Geometry: final body of the model. Coordinates: model frame, mm. Coordinates: 2 decimals unless noted, no trailing zeros. Order: outer loops, then holes, each group sorted by start corner. A loop starts at its lowest first (then second) coordinate and runs counter-clockwise, first axis right, second up. Notation, with made-up numbers: (71, 12) -> (88, 12) arc R33 cw to (88, 44) -> close; hole circle Ø9 at (1.5, -38.5). An arc over 180 degrees is marked (long way). Use one line per item in the form item = value.
```python
from build123d import *

# Parameters (mm, degrees)
SKETCH_1_W      = 23
SKETCH_1_H      = 4.3
EXTRUDE_1_DEPTH = 0.6


with BuildPart() as part:
    # Эскиз1 → Бобышка-Вытянуть1 (new body)
    with BuildSketch(Plane.XY):
        with BuildLine():
            Line((0, 0), (56, 0))
            Line((56, 0), (56, 15.7))
            Line((56, 15.7), (15, 15.7))
            ThreePointArc((15, 15.7), (10.112556238, 5.353927161), (0, 0))
        make_face()
        with Locations((37.5, 7.85)):
            Rectangle(SKETCH_1_W, SKETCH_1_H, mode=Mode.SUBTRACT)
    extrude(amount=EXTRUDE_1_DEPTH)


solid = part.part
```
1) Section C-C, the plane y = 7. Output: boundary loops of the cut face in (x, z), and give its area (3 significant figures).
Results found:
outline = (11.51, 0) -> (26, 0) -> (26, 0.6) -> (11.51, 0.6) -> close; (49, 0) -> (56, 0) -> (56, 0.6) -> (49, 0.6) -> close
area = 12.9 mm2
2) Section A-A, the plane z = 0.5. Output: boundary loops of the cut face in (x, y).
Results found:
outline = (0, 0) -> (56, 0) -> (56, 15.7) -> (15, 15.7) arc R18.12 cw to start; hole (26, 5.7) -> (49, 5.7) -> (49, 10) -> (26, 10) -> close
3) Material intervals for probe 1 along Y at (x, z) = (38.5, 0.4); probe 2 along X at (y, z) = (8.75, 0.4); probe 3 along Y at (x, z) = (13, 0.1), sorted ascending. Write a range as from..to.
Results found:
probe_1 = 0..5.7, 10..15.7
probe_2 = 12.67..26, 49..56
probe_3 = 0..9.35
4) Section B-B, the plane x = 35. Output: boundary loops of the cut face in (y, z).
Results found:
outline = (0, 0) -> (5.7, 0) -> (5.7, 0.6) -> (0, 0.6) -> close; (10, 0) -> (15.7, 0) -> (15.7, 0.6) -> (10, 0.6) -> close
5) Section D-D, the plane x = 5.5. Output: boundary loops of the cut face in (y, z), and give its area (3 significant figures).
Results found:
outline = (0, 0) -> (1.86, 0) -> (1.86, 0.6) -> (0, 0.6) -> close
area = 1.12 mm2
